The listing builds one solid part. Answer for the finished solid, in the listing's coordinates (mm). A direction names the side the tool comes from. Coordinates: 2 decimals unless noted, no trailing zeros. Write each loop counter-clockwise with the first axis right and the second up, starting at its lowest first coordinate (ties: lowest second). Pieces come first, ordered by that corner, then holes.
from build123d import *

# Parameters (mm, degrees)
SKETCH1_W           = 110
SKETCH1_H           = 130
BOSS_EXTRUDE1_DEPTH = 5
SKETCH10_W          = 110
SKETCH10_H          = 60
BOSS_EXTRUDE4_DEPTH = 13
SKETCH6_R           = 21
CUT_EXTRUDE2_DEPTH  = 30
BOSS_EXTRUDE6_START = 12
SKETCH16_R          = 27.5
SKETCH16_R_2        = 21
BOSS_EXTRUDE6_DEPTH = 12
BOSS_EXTRUDE7_START = 5
SKETCH17_R          = 27.5
SKETCH17_R_2        = 10
BOSS_EXTRUDE7_DEPTH = 5
BOSS_EXTRUDE8_DEPTH = 50
SKETCH19_R          = 10
CUT_EXTRUDE3_DEPTH  = 50
SKETCH21_R          = 21
CUT_EXTRUDE4_DEPTH  = 12
BOSS_EXTRUDE9_START = 8
SKETCH22_R          = 22.5
SKETCH22_R_2        = 10
BOSS_EXTRUDE9_DEPTH = 8
FILLET1_R           = 10
FILLET2_R           = 10
FILLET3_R           = 2
SKETCH23_R          = 13
CUT_EXTRUDE5_DEPTH  = 9
SKETCH24_R          = 5
CUT_EXTRUDE6_DEPTH  = 9
SKETCH27_R          = 2
CUT_EXTRUDE7_DEPTH  = 10
SKETCH28_R          = 2
CUT_EXTRUDE8_DEPTH  = 10


with BuildPart() as part:
    # Sketch1 → Boss-Extrude1 (new, symmetric)
    with BuildSketch(Plane.XY):
        with Locations((0, 5)):
            Rectangle(SKETCH1_W, SKETCH1_H)
    extrude(amount=BOSS_EXTRUDE1_DEPTH, both=True)

    # Sketch10 → Boss-Extrude4 (add)
    with BuildSketch(Plane.XZ.offset(60)):
        with Locations((0, 25)):
            Rectangle(SKETCH10_W, SKETCH10_H)
    extrude(amount=-BOSS_EXTRUDE4_DEPTH)

    # Sketch6 → Cut-Extrude2 (cut)
    with BuildSketch(Plane(origin=(0, 0, -5), x_dir=(-1, 0, 0), z_dir=(0, 0, -1))):
        with Locations((0, 20)):
            Circle(SKETCH6_R)
    extrude(amount=-CUT_EXTRUDE2_DEPTH, mode=Mode.SUBTRACT)

    # Sketch16 → Boss-Extrude6 (add)
    with BuildSketch(Plane(origin=(0, 0, -5), x_dir=(-1, 0, 0), z_dir=(0, 0, -1)).offset(BOSS_EXTRUDE6_START)):
        with Locations((0, 20)):
            Circle(SKETCH16_R)
        with Locations((0, 20)):
            Circle(SKETCH16_R_2, mode=Mode.SUBTRACT)
    extrude(amount=-BOSS_EXTRUDE6_DEPTH)

    # Sketch17 → Boss-Extrude7 (add)
    with BuildSketch(Plane(origin=(0, 0, -17), x_dir=(-1, 0, 0), z_dir=(0, 0, -1)).offset(BOSS_EXTRUDE7_START)):
        with Locations((0, 20)):
            Circle(SKETCH17_R)
        with Locations((0, 20)):
            Circle(SKETCH17_R_2, mode=Mode.SUBTRACT)
    extrude(amount=-BOSS_EXTRUDE7_DEPTH)

    # Sketch18 → Boss-Extrude8 (add)
    with BuildSketch(Plane.XY.offset(5)):
        with BuildLine():
            Line((-55, -47), (-39, -47))
            Line((-39, -47), (-39, -17.822222222))
            Line((-39, -17.822222222), (-30.482216757, -17.822222222))
            Line((-30.482216757, -17.822222222), (-30.482216757, -14.450463881))
            ThreePointArc((-30.482216757, -14.450463881), (0, 66), (30.482216757, -14.450463881))
            Line((30.482216757, -14.450463881), (30.482216757, -17.822222222))
            Line((30.482216757, -17.822222222), (39, -17.822222222))
            Line((39, -17.822222222), (39, -47))
            Line((39, -47), (55, -47))
            Line((55, -47), (55, 70))
            Line((55, 70), (-55, 70))
            Line((-55, 70), (-55, -47))
        make_face()
    extrude(amount=BOSS_EXTRUDE8_DEPTH)

    # Sketch19 → Cut-Extrude3 (cut)
    with BuildSketch(Plane.XZ.offset(60)):
        with Locations(Location((0, 25, 0), (0, 0, 270))):
            Circle(SKETCH19_R)
    extrude(amount=-CUT_EXTRUDE3_DEPTH, mode=Mode.SUBTRACT)

    # Sketch21 → Cut-Extrude4 (cut)
    with BuildSketch(Plane(origin=(0, -47, 0), x_dir=(1, 0, 0), z_dir=(0, 1, 0))):
        with Locations(Location((0, -25, 0), (0, 0, 270))):
            Circle(SKETCH21_R)
    extrude(amount=-CUT_EXTRUDE4_DEPTH, mode=Mode.SUBTRACT)

    # Sketch22 → Boss-Extrude9 (add)
    with BuildSketch(Plane.XZ.offset(60).offset(BOSS_EXTRUDE9_START)):
        with Locations(Location((0, 25, 0), (0, 0, 270))):
            Circle(SKETCH22_R)
        with Locations(Location((0, 25, 0), (0, 0, 270))):
            Circle(SKETCH22_R_2, mode=Mode.SUBTRACT)
    extrude(amount=-BOSS_EXTRUDE9_DEPTH)

    # Fillet1
    # the kernel refuses this fillet: 10 mm, written as the material it adds along each edge
    with BuildSketch(Plane(origin=(0, -60, 25), x_dir=(0, 0, -1), z_dir=(-1, 0, 0))) as fillet1_piece_1_section:
        with BuildLine():
            CenterArc((32.297958971, 10), FILLET1_R, 191.536959033, 78.463040967)
            Line((22.5, 8), (22.5, 0))
            Line((22.5, 0), (32.297958971, 0))
        make_face()
    fillet1_piece_1 = revolve(axis=Axis((0, -60, 25), (0, -1, 0)), mode=Mode.PRIVATE)
    fillet1_piece_1 = split(fillet1_piece_1, bisect_by=Plane(origin=(0, -60, 55), z_dir=(0, 0, -1)), keep=Keep.TOP, mode=Mode.PRIVATE)
    fillet1_piece_1 = split(fillet1_piece_1, bisect_by=Plane(origin=(0, -60, -5), z_dir=(0, 0, 1)), keep=Keep.TOP, mode=Mode.PRIVATE)
    add(fillet1_piece_1)

    # Fillet2
    fillet2_edges = [part.edges().sort_by_distance(p)[0] for p in [
        (27.5, 20, -5),
    ]]
    fillet(fillet2_edges, radius=FILLET2_R)

    # Fillet3
    fillet3_edges = [part.edges().sort_by_distance(p)[0] for p in [
        (27.5, 20, -22),
    ]]
    fillet(fillet3_edges, radius=FILLET3_R)

    # Sketch23 → Cut-Extrude5 (cut)
    with BuildSketch(Plane(origin=(-39, 0, 0), x_dir=(0, 0, -1), z_dir=(1, 0, 0))):
        with Locations((-25, -32)):
            Circle(SKETCH23_R)
    cut_extrude5 = extrude(amount=-CUT_EXTRUDE5_DEPTH, mode=Mode.SUBTRACT)

    # Sketch24 → Cut-Extrude6 (cut)
    with BuildSketch(Plane(origin=(-48, 0, 0), x_dir=(0, 0, -1), z_dir=(1, 0, 0))):
        with Locations((-25, -32)):
            Circle(SKETCH24_R)
    cut_extrude6 = extrude(amount=-CUT_EXTRUDE6_DEPTH, mode=Mode.SUBTRACT)

    # Mirror1: Cut-Extrude5, Cut-Extrude6 across plane
    add(cut_extrude5.mirror(Plane(origin=(0, 0, 0), x_dir=(0, 0, 1), z_dir=(1, 0, 0))), mode=Mode.SUBTRACT)
    add(cut_extrude6.mirror(Plane(origin=(0, 0, 0), x_dir=(0, 0, 1), z_dir=(1, 0, 0))), mode=Mode.SUBTRACT)

    # Sketch27 → Cut-Extrude7 (cut)
    with BuildSketch(Plane.ZY.offset(55)):
        with Locations((2, -32)):
            Circle(SKETCH27_R)
        with Locations(Location((48, -32, 0), (0, 0, 180))):
            Circle(SKETCH27_R)
        with Locations((25, -55)):
            Circle(SKETCH27_R)
        with Locations(Location((25, -9, 0), (0, 0, 180))):
            Circle(SKETCH27_R)
    cut_extrude7 = extrude(amount=-CUT_EXTRUDE7_DEPTH, mode=Mode.SUBTRACT)

    # Mirror2: Cut-Extrude7 across plane
    add(cut_extrude7.mirror(Plane(origin=(0, 0, 0), x_dir=(0, 0, 1), z_dir=(1, 0, 0))), mode=Mode.SUBTRACT)

    # Sketch28 → Cut-Extrude8 (cut)
    with BuildSketch(Plane.XY.offset(55)):
        with Locations((-45, 60)):
            Circle(SKETCH28_R)
        with Locations((-45, -12)):
            Circle(SKETCH28_R)
        with Locations((-47, -52)):
            Circle(SKETCH28_R)
        with Locations(Location((47, -52, 0), (0, 0, 180))):
            Circle(SKETCH28_R)
        with Locations(Location((45, -12, 0), (0, 0, 180))):
            Circle(SKETCH28_R)
        with Locations(Location((45, 60, 0), (0, 0, 180))):
            Circle(SKETCH28_R)
    extrude(amount=-CUT_EXTRUDE8_DEPTH, mode=Mode.SUBTRACT)


solid = part.part
Q1. Determine the mould class of faces 1 (the face through (-45, -32, 48)), 2 (the face through (-1, -47, 47)), 3 (the face through (-50.07, -10.352, 26.474)) for opening direction X: released by +X, released by -X, zero draft, split by the parting line, or undercut.
Answers below:
face 1: released by -X
face 2: undercut
face 3: zero draft
Q2. The part is cut by section C-C, the plane x = -8. State how many separate pieces and enclosed holes the cut face has, then the cut area to 3 significant figures.
Answers below:
separate pieces: 3
enclosed holes: 0
area: 2,010 mm2
Q3. Given pin 1 (3 mm diameter, centred on x = -45, y = -12, fed in from +Z); pin 2 (1 mm diameter, centred on x = 15, z = 4, fed in from -Y); pin 3 (10 mm diameter, centred on x = 20, y = -47.5, fed in from -Z), each flat-ended and moving along its own axis, determine where each tip first touches the part or whether it passes through.
Answers below:
pin 1: stops at z = 45
pin 2: stops at y = -62.85
pin 3: stops at z = -5
Q4. The part is cut by section A-A, the plane z = -9. Write down the section's boundary in (x, y).
Answers below:
outline: circle Ø59 at (0, 20); hole circle Ø42 at (0, 20)
Q5. Which of the six approach directions +Z, -Z, +X, -X, +Y, -Y give full straight-line access (tool end or side, diameter ignored) to faces 4 (the face through (50.07, -10.352, 26.474)), 5 (the face through (3, -63.56, 15.46)), 6 (the face through (-43.44, -21.04, 18.01)), 7 (the face through (-9, 25, -17)), 8 (the face through (-50, -30, 48))?
Answers below:
face 4: +X
face 5: -Y
face 6: none
face 7: +Z
face 8: -X
Q6. The part is cut by section B-B, the plane y = 60. Write down the section's boundary in (x, z), then the cut area to 3 significant figures.
Answers below:
outline: (-55, -5) - (55, -5) - (55, 55) - (47, 55) - (47, 45) - (43, 45) - (43, 55) - (22.72, 55) - (22.72, 5) - (-22.72, 5) - (-22.72, 55) - (-43, 55) - (-43, 45) - (-47, 45) - (-47, 55) - (-55, 55) - close
area: 4,250 mm2
Q7. Find the intervals of material crossed by probe 1 along Y at (x, z) = (53, 25); probe 2 along Y at (x, z) = (-42.5, 25); probe 3 along X at (y, z) = (-19, 14), in increasing order.
Answers below:
probe 1: y = -60 to -57, -53 to -37, -27 to -11, -7 to 70
probe 2: y = -60 to -45, -19 to 2.4, 37.6 to 70
probe 3: x = -55 to -39, 39 to 55
